```python
from build123d import *

# Parameters (mm, degrees)
F2_R     = 13.85
F3_DEPTH = 17.501
F4_R     = 7.95
F5_DEPTH = 15.901


with BuildPart() as f1:
    # F0 (on Front) → F1 (revolve)
    with BuildSketch(Plane.XZ):
        with BuildLine():
            Line((-21.45, 0), (0, 0))
            Line((0, 0), (0, 17.5))
            Line((0, 17.5), (-18.485754, 17.5))
            Line((-18.485754, 17.5), (-19.05, 14.3))
            Line((-19.05, 14.3), (-47.2, 14.3))
            ThreePointArc((-47.2, 14.3), (-48.614214, 13.714214), (-49.2, 12.3))
            Line((-49.2, 12.3), (-49.2, 1.6))
            Line((-49.2, 1.6), (-21.45, 1.6))
            Line((-21.45, 1.6), (-21.45, 0))
        make_face()
    revolve(axis=Axis((0, 0, 8.75), (0, 0, -1)))

    # F2 (on face) → F3 (cut, through all)
    with BuildSketch(Plane(origin=(0, 0, 0), x_dir=(1, 0, 0), z_dir=(0, 0, -1))):
        Circle(F2_R)
    extrude(amount=-F3_DEPTH, mode=Mode.SUBTRACT)

    # F4 (on face) → F5 (cut, through all)
    with BuildSketch(Plane(origin=(0, 0, 1.6), x_dir=(1, 0, 0), z_dir=(0, 0, -1))):
        with Locations((0, 34.9)):
            Circle(F4_R)
        with Locations((-34.9, 0)):
            Circle(F4_R)
        with Locations((0, -34.9)):
            Circle(F4_R)
        with Locations((34.9, 0)):
            Circle(F4_R)
    extrude(amount=-F5_DEPTH, mode=Mode.SUBTRACT)


solid = f1.part
```
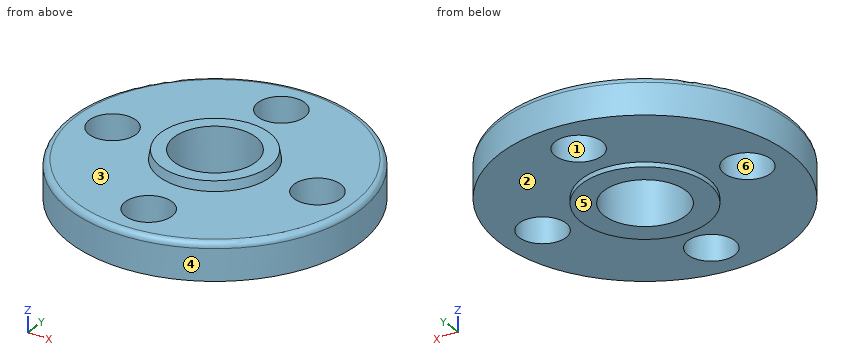
Geometry: final body of the model. Coordinates: model frame, mm. Face numbers are marked on the shaded views. A direction names the side the tool comes from. Round coordinates to 2 decimals unless told otherwise and drop trailing zeros. Order: outer loops, then holes, each group sorted by start corner. A loop starts at its lowest first (then second) coordinate and runs counter-clockwise, first axis right, second up. Notation, with made-up numbers: (14.5, 44.25) - (69.5, 44.25) arc R22 ccw to (69.5, 64.25) - close; hole circle Ø11 at (22.5, 60). An arc over 180 degrees is marked (long way). Use CSV: the item, a comma, the result in double quotes. Start each with the question number.
Q1. Mould query, pull axis Y, two halves, no side actions, for the marked faces 4, 5 and 6. Classes: +Y half, -Y half, draft (parallel to the pull), parting line (faces both ways), or undercut.
Q2. Material intervals for line 1 along Y through (x, z) = (0, 9.5); line 2 along Y through (x, z) = (-1.5, 2); line 3 along Z through (x, y) = (-11, 24.5), sorted ascending. Write a range as from..to.
Q3. First-contact query: pin 1 (2 mm diameter, centred on x = 24, y = -5, fed in from -Z); pin 2 (14.5 mm diameter, centred on x = 0, y = 34.9, fed in from +Z); pin 3 (12 mm diameter, centred on x = 11, y = 16.5, fed in from +Z); pin 4 (1.5 mm diameter, centred on x = -13, y = 23.5, fed in from +Z). Flat tips, straight axial feed; report the tip coordinate or a pass-through.
Q4. Section query A-A (x = 0). Return loops of the section in (y, z).
Q5. Access query for the marked faces 1, 2 and 3. Directions: +Z, -Z, +X, -X, +Y, -Y. A direction counts if a zero-diameter tool reaches every point of the face in a straight line with its end or side. Return the directions, or none.
Q6. Section query B-B (z = 15.75). Return loops of the section in (x, y), and give its area (3 significant figures).
Result set:
1,face 4,"parting line"
1,face 5,"draft"
1,face 6,"undercut"
2,line 1,"y = -49.2..-42.85, -26.95..-13.85, 13.85..26.95, 42.85..49.2"
2,line 2,"y = -49.18..-42.71, -27.09..-13.77, 13.77..27.09, 42.71..49.18"
2,line 3,"z = 1.6..14.3"
3,pin 1,"stops at z = 1.6"
3,pin 2,"passes through"
3,pin 3,"stops at z = 17.5"
3,pin 4,"stops at z = 14.3"
4,outline,"(-49.2, 1.6) - (-42.85, 1.6) - (-42.85, 14.3) - (-47.2, 14.3) arc R2 ccw to (-49.2, 12.3) - close; (-26.95, 1.6) - (-21.45, 1.6) - (-21.45, 0) - (-13.85, 0) - (-13.85, 17.5) - (-18.49, 17.5) - (-19.05, 14.3) - (-26.95, 14.3) - close; (13.85, 0) - (21.45, 0) - (21.45, 1.6) - (26.95, 1.6) - (26.95, 14.3) - (19.05, 14.3) - (18.49, 17.5) - (13.85, 17.5) - close; (42.85, 1.6) - (49.2, 1.6) - (49.2, 12.3) arc R2 ccw to (47.2, 14.3) - (42.85, 14.3) - close"
5,face 1,"+Z, -Z"
5,face 2,"-Z"
5,face 3,"+Z"
6,outline,"circle Ø37.59 at (0, 0); hole circle Ø27.7 at (0, 0)"
6,area,"507 mm2"
